```python
from build123d import *

# Parameters (mm, degrees)
EXTRUDE1_DEPTH = 6.35


with BuildPart() as part:
    # Sketch1 → Extrude1 (new body)
    with BuildSketch(Plane.XY):
        Polygon((500.815587146, 387.589172699), (500.815587146, 19.289172699), (469.065587146, 19.289172699), (469.065587146, 25.639172699), (443.665587146, 25.639172699), (443.665587146, 19.289172699), (418.265587146, 19.289172699), (418.265587146, 25.639172699), (392.865587146, 25.639172699), (392.865587146, 19.289172699), (367.465587146, 19.289172699), (367.465587146, 25.639172699), (342.065587146, 25.639172699), (342.065587146, 19.289172699), (329.365587146, 19.289172699), (329.365587146, 25.639172699), (303.965587146, 25.639172699), (303.965587146, 19.289172699), (291.265587146, 19.289172699), (291.265587146, 25.639172699), (265.865587146, 25.639172699), (265.865587146, 19.289172699), (240.465587146, 19.289172699), (240.465587146, 25.639172699), (215.065587146, 25.639172699), (215.065587146, 19.289172699), (189.665587146, 19.289172699), (189.665587146, 25.639172699), (164.265587146, 25.639172699), (164.265587146, 19.289172699), (132.515587146, 19.289172699), (132.515587146, 51.039172699), (138.865587146, 51.039172699), (138.865587146, 76.439172699), (132.515587146, 76.439172699), (132.515587146, 101.839172699), (138.865587146, 101.839172699), (138.865587146, 127.239172699), (132.515587146, 127.239172699), (132.515587146, 152.639172699), (138.865587146, 152.639172699), (138.865587146, 178.039172699), (132.515587146, 178.039172699), (132.515587146, 190.739172699), (138.865587146, 190.739172699), (138.865587146, 216.139172699), (132.515587146, 216.139172699), (132.515587146, 228.839172699), (138.865587146, 228.839172699), (138.865587146, 254.239172699), (132.515587146, 254.239172699), (132.515587146, 279.639172699), (138.865587146, 279.639172699), (138.865587146, 305.039172699), (132.515587146, 305.039172699), (132.515587146, 330.439172699), (138.865587146, 330.439172699), (138.865587146, 355.839172699), (132.515587146, 355.839172699), (132.515587146, 387.589172699), (164.265587146, 387.589172699), (164.265587146, 381.239172699), (189.665587146, 381.239172699), (189.665587146, 387.589172699), (215.065587146, 387.589172699), (215.065587146, 381.239172699), (240.465587146, 381.239172699), (240.465587146, 387.589172699), (265.865587146, 387.589172699), (265.865587146, 381.239172699), (291.265587146, 381.239172699), (291.265587146, 387.589172699), (303.965587146, 387.589172699), (303.965587146, 381.239172699), (329.365587146, 381.239172699), (329.365587146, 387.589172699), (342.065587146, 387.589172699), (342.065587146, 381.239172699), (367.465587146, 381.239172699), (367.465587146, 387.589172699), (392.865587146, 387.589172699), (392.865587146, 381.239172699), (418.265587146, 381.239172699), (418.265587146, 387.589172699), (443.665587146, 387.589172699), (443.665587146, 381.239172699), (469.065587146, 381.239172699), (469.065587146, 387.589172699), align=None)
    extrude(amount=EXTRUDE1_DEPTH)


solid = part.part
```
Check sheet for the modelled part. Datum: model origin and axes. Units: mm. Coordinates: 2 decimals unless noted, no trailing zeros. Order: outer loops, then holes, each group sorted by start corner. A loop starts at its lowest first (then second) coordinate and runs counter-clockwise, first axis right, second up. Notation, with made-up numbers: M 32,46 L 59,46 A19 cw 59,79 Z; hole C 55.5,64 d1. An arc over 180 degrees is marked long. One line per question, with ' | ' between items. Start each with the question number.
Item 1: Material ranges on line 1 (Y direction, x = 173.5, z = 3); line 2 (X direction, y = 301, z = 2.5), recorded low to high.
Item 2: Gauge pin test, flat ends, axial feed: P1, Ø1.9, axis at y = 117.5, z = 2, coming from the -X side; P2, Ø8, axis at x = 214.5, y = 136.5, coming from the -Z side; P3, Ø3, axis at x = 318.5, z = 3.5, coming from the -Y side. Record the tip position at first contact, or that the pin passes through.
Item 3: Sectioned sample at A-A on x = 404.5. Record the cut outline in (y, z).
Item 4: Sectioned sample at B-B on y = 169. Record the cut outline in (x, z).
Answer below:
1) line 1: y = 25.64 to 381.24 | line 2: x = 138.87 to 500.82
2) P1: stops at x = 138.87 | P2: stops at z = 0 | P3: stops at y = 25.64
3) outline: M 25.64,0 L 381.24,0 L 381.24,6.35 L 25.64,6.35 Z
4) outline: M 138.87,0 L 500.82,0 L 500.82,6.35 L 138.87,6.35 Z
